```python
from build123d import *

# Parameters (mm, degrees)
SKETCH1_R           = 15
BOSS_EXTRUDE1_DEPTH = 30
SKETCH2_R           = 20
CUT_EXTRUDE1_DEPTH  = 16
BOSS_EXTRUDE2_DEPTH = 35
CUT_EXTRUDE3_DEPTH  = 51


with BuildPart() as part:
    # Sketch1 → Boss-Extrude1 (new body, symmetric)
    with BuildSketch(Plane.XY):
        with BuildLine():
            Line((25, 0), (25, 80))
            Line((25, 80), (10, 80))
            Line((10, 80), (10, 22.912878475))
            Line((10, 22.912878475), (10, 20))
            Line((10, 20), (-25, 20))
            Line((-25, 20), (-25, 0))
            ThreePointArc((-25, 0), (0, -25), (25, 0))
        make_face()
        Circle(SKETCH1_R, mode=Mode.SUBTRACT)
    extrude(amount=BOSS_EXTRUDE1_DEPTH, both=True)

    # Sketch2 → Cut-Extrude1 (cut, through all)
    with BuildSketch(Plane.ZY.offset(-10)):
        with Locations((0, 80)):
            Circle(SKETCH2_R)
    extrude(amount=-CUT_EXTRUDE1_DEPTH, mode=Mode.SUBTRACT)

    # Sketch4 → Boss-Extrude2 (add)
    with BuildSketch(Plane.ZY.offset(25)):
        with BuildLine():
            Line((-15, 20), (-30, 20))
            ThreePointArc((-30, 20), (0, 50), (30, 20))
            Line((30, 20), (15, 20))
            ThreePointArc((15, 20), (0, 35), (-15, 20))
        make_face()
    extrude(amount=-BOSS_EXTRUDE2_DEPTH)

    # Sketch5 → Cut-Extrude3 (cut, through all)
    with BuildSketch(Plane.ZY.offset(25)):
        with BuildLine():
            Line((-15, 19.774418989), (-15, -47.367007727))
            Line((-15, -47.367007727), (15.001696131, -47.367007727))
            Line((15.001696131, -47.367007727), (15.001696131, -44.584519051))
            Line((15.001696131, -44.584519051), (15.001696131, 20))
            ThreePointArc((15.001696131, 20), (-0.112793694, 35.001272092), (-15, 19.774418989))
        make_face()
    extrude(amount=-CUT_EXTRUDE3_DEPTH, mode=Mode.SUBTRACT)


solid = part.part
```
Model file for the job. Use its own axes, mm. A direction names the side the tool comes from. Coordinates: 2 decimals unless noted, no trailing zeros. Loops run counter-clockwise (first coordinate to the right, second up) from the corner with the lowest first, then second, coordinate; pieces in that order, holes last. Notation, with made-up numbers: (45, 54) - (58, 54) arc R29 ccw to (58, 74) - close; hole circle Ø2 at (56, -27). An arc over 180 degrees is marked (long way). Answer as a JSON object with one key per item and string values. Group by question number.
(1) Cut at A-A (y = 17). Give the cut face in (x, z), then the cut area to 3 significant figures.
(2) Cut at C-C (y = 6). Give the cut face in (x, z), then the cut area to 3 significant figures.
(3) Tool access for faces 4 (the face through (-7.745, 49.993, -0.66)), 5 (the face through (-11, -13, 15.002)), 6 (the face through (-0.55, -24.994, -22.395)): list every direction of +Z, -Z, +X, -X, +Y, -Y with a clear straight run to the whole face (end or side of a thin tool).
(4) Cut at D-D (z = 26). Give the cut face in (x, y).
(5) Probe line 1 along Z through (x, y) = (18.5, -2); line 2 along X through (y, z) = (0, -26.5); line 3 along Y through (x, z) = (-9, -18). List the from-to ranges inside material, lowest first.
(6) Cut at B-B (x = 0). Give the cut face in (y, z), then the cut area to 3 significant figures.
(7) Flat gauge pins, fed straight in: pin 1 (1 mm diameter, centred on y = -6.5, z = 20, fed in from +X); pin 2 (2 mm diameter, centred on x = -7.5, y = 21, fed in from -Z); pin 3 (1.5 mm diameter, centred on y = 45, z = -20.5, fed in from -X); pin 4 (10 mm diameter, centred on x = 0, z = -9.5, fed in from +Y). Where does each tip first touch, or does it go through?
(8) Two-plate mould, pull along Y, no slides. Class faces 1 (the face through (-14.985, 0.66, -22.605)), 2 (the face through (17, 60, 0)), 3 (the face through (10, 57, 0)): released by +Y, released by -Y, zero draft, split by the parting line, or undercut.
Geometry says:
{
 "1": {"outline": "(-25, -30) - (25, -30) - (25, -15) - (-25, -15) - close; (-25, 15) - (25, 15) - (25, 30) - (-25, 30) - close", "area": "1,500 mm^2"},
 "2": {"outline": "(-25, -30) - (-13.75, -30) - (-13.75, -15) - (-25, -15) - close; (-25, 15) - (-13.75, 15) - (-13.75, 30) - (-25, 30) - close; (13.75, -30) - (25, -30) - (25, -15) - (13.75, -15) - close; (13.75, 15) - (25, 15) - (25, 30) - (13.75, 30) - close", "area": "675 mm^2"},
 "3": {"face 4": "-X, +Y", "face 5": "+X, -X, -Y", "face 6": "+Z, -Z, -Y"},
 "4": {"outline": "(-25, 0) arc R25 ccw to (25, 0) - (25, 80) - (10, 80) - (10, 34.97) - (-25, 34.97) - close; hole circle Ø30 at (0, 0)"},
 "5": {"line 1": "z = -30 to -15, 15 to 30", "line 2": "x = -25 to -15, 15 to 25", "line 3": "y = -23.32 to -12, 12 to 44"},
 "6": {"outline": "(-25, -30) - (-15, -30) - (-15, -15) - (-25, -15) - close; (-25, 15) - (-15, 15) - (-15, 30) - (-25, 30) - close; (15, -30) - (20, -30) arc R30 ccw to (20, 30) - (15, 30) - (15, 15) - (20, 15) arc R15 cw (long way) to (19.77, -15) - (15, -15) - close", "area": "1,510 mm^2"},
 "7": {"pin 1": "stops at x = 24.27", "pin 2": "stops at z = -30", "pin 3": "stops at x = 10", "pin 4": "stops at y = 49.66"},
 "8": {"face 1": "undercut", "face 2": "released by +Y", "face 3": "zero draft"}
}
